```python
from build123d import *

# Parameters (mm, degrees)
F1_DEPTH = 27
F2_DEPTH = 2


with BuildPart() as f1:
    # F0 (on Top) → F1 (new body)
    with BuildSketch(Plane.XY):
        with BuildLine():
            Line((-52.5, 5.5), (-55, 5.5))
            ThreePointArc((-55, 5.5), (-60.5, 0), (-55, -5.5))
            Line((-55, -5.5), (-52.5, -5.5))
            ThreePointArc((-52.5, -5.5), (-48.982188, -4.227884), (-47.091673, -1))
            ThreePointArc((-47.091673, -1), (-47, 0), (-47.091673, 1))
            ThreePointArc((-47.091673, 1), (-48.982188, 4.227884), (-52.5, 5.5))
        make_face()
        with BuildLine():
            ThreePointArc((-52.5, 4.5), (-48, 0), (-52.5, -4.5))
            Line((-52.5, -4.5), (-55, -4.5))
            ThreePointArc((-55, -4.5), (-59.5, 0), (-55, 4.5))
            Line((-55, 4.5), (-52.5, 4.5))
        make_face(mode=Mode.SUBTRACT)
    extrude(amount=F1_DEPTH)

    # F0 (on Top) → F2 (join)
    with BuildSketch(Plane.XY):
        with BuildLine():
            Line((0, 1), (-47.091673, 1))
            ThreePointArc((-47.091673, 1), (-47, 0), (-47.091673, -1))
            Line((-47.091673, -1), (0, -1))
            Line((0, -1), (0, 1))
        make_face()
    extrude(amount=F2_DEPTH)

    # F3: F1 across plane


with BuildPart() as f1_1:
    add(f1.part)
    add(f1.part.mirror(Plane.YZ))


solid = f1_1.part
```
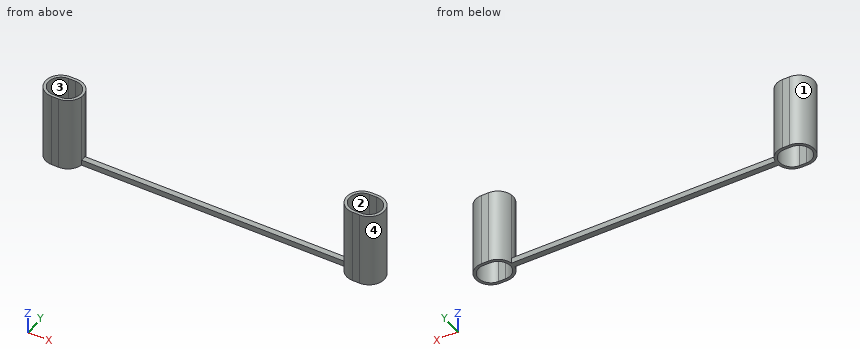
The listing builds one solid part. Answer for the finished solid, in the listing's coordinates (mm). Face numbers are marked on the shaded views. A direction names the side the tool comes from. Round coordinates to 2 decimals unless told otherwise and drop trailing zeros. Write each loop counter-clockwise with the first axis right and the second up, starting at its lowest first coordinate (ties: lowest second). Pieces come first, ordered by that corner, then holes. Notation, with made-up numbers: (74.5, 40.25) -> (90.5, 40.25) arc R26 ccw to (90.5, 75.25) -> close; hole circle Ø5 at (41, 59). An arc over 180 degrees is marked (long way). Write item = value, one per line.
1) For a pull along Y with two mould halves and no side action, classify the marked faces 1 and 2 as released by +Y, released by -Y, zero draft, split by the parting line, or undercut.
Check values:
face_1 = split by the parting line
face_2 = undercut
2) Section A-A on z = 6.5 is taken. Write down the section's boundary in (x, y), plus the area to 3 significant figures.
Check values:
outline = (-55, -5.5) -> (-52.5, -5.5) arc R5.5 ccw to (-47.09, -1) arc R5.5 ccw to (-47.09, 1) arc R5.5 ccw to (-52.5, 5.5) -> (-55, 5.5) arc R5.5 ccw to start; (47.09, -1) arc R5.5 ccw to (52.5, -5.5) -> (55, -5.5) arc R5.5 ccw to (55, 5.5) -> (52.5, 5.5) arc R5.5 ccw to (47.09, 1) arc R5.5 ccw to start; hole (-55, -4.5) -> (-52.5, -4.5) arc R4.5 ccw to (-52.5, 4.5) -> (-55, 4.5) arc R4.5 ccw to start; hole (52.5, -4.5) -> (55, -4.5) arc R4.5 ccw to (55, 4.5) -> (52.5, 4.5) arc R4.5 ccw to start
area = 72.8 mm²
3) Given pin 1 (2 mm diameter, centred on x = -10, z = 1, fed in from -Y); pin 2 (0.6 mm diameter, centred on x = -22.5, y = 0, fed in from +Z); pin 3 (1.5 mm diameter, centred on y = -1.5, z = 5.5, fed in from +X), each flat-ended and moving along its own axis, determine where each tip first touches the part or whether it passes through.
Check values:
pin_1 = -1
pin_2 = 2
pin_3 = 60.45
4) Which of the six approach directions +Z, -Z, +X, -X, +Y, -Y give full straight-line access (tool end or side, diameter ignored) to the marked faces 3 and 4?
Check values:
face_3 = +Z, -Z
face_4 = +Z, -Z, +X
5) Section C-C on x = 40.5 is taken. Write down the section's boundary in (y, z), plus the area to 3 significant figures.
Check values:
outline = (-1, 0) -> (1, 0) -> (1, 2) -> (-1, 2) -> close
area = 4.00 mm²
6) Straight lines are drawn through the part: line 1 along X through (y, z) = (0, 14); line 2 along X through (y, z) = (3.25, 24.75); line 3 along X through (y, z) = (4.75, 17.5). For each, find the intervals that lie inside material, in ascending order. Write a range as [from, to].
Check values:
line_1 = [-60.5, -59.5], [-48, -47], [47, 48], [59.5, 60.5]
line_2 = [-59.44, -58.11], [-49.39, -48.06], [48.06, 49.39], [58.11, 59.44]
line_3 = [-57.77, -49.73], [49.73, 57.77]
7) Section B-B on y = 0 is taken. Write down the section's boundary in (x, z), plus the area to 3 significant figures.
Check values:
outline = (-60.5, 0) -> (-59.5, 0) -> (-59.5, 27) -> (-60.5, 27) -> close; (-48, 0) -> (48, 0) -> (48, 27) -> (47, 27) -> (47, 2) -> (-47, 2) -> (-47, 27) -> (-48, 27) -> close; (59.5, 0) -> (60.5, 0) -> (60.5, 27) -> (59.5, 27) -> close
area = 296 mm²
